Design review of the part built by this model. Coordinates are the model's own, in mm. Face numbers are marked on the shaded views. Give positions to 0.01 mm unless a question says otherwise; leave off trailing zeros. Order: outer loops, then holes, each group sorted by start corner. A loop starts at its lowest first (then second) coordinate and runs counter-clockwise, first axis right, second up. Notation, with made-up numbers: (66, 25.5) -> (102, 25.5) arc R9 cw to (102, 36.5) -> close; hole circle Ø8 at (10, 1.25). An arc over 180 degrees is marked (long way). One line per item, written item: value.
from build123d import *

# Parameters (mm, degrees)
F1_DEPTH = 25
F2_R     = 6
F2_R_2   = 8.25
F3_DEPTH = 20


with BuildPart() as f1:
    # F0 (on Top) → F1 (new body)
    with BuildSketch(Plane.XY):
        with BuildLine():
            Line((-58.75, -42.5), (58.75, -42.5))
            ThreePointArc((58.75, -42.5), (62.285534, -41.035534), (63.75, -37.5))
            Line((63.75, -37.5), (63.75, 37.5))
            ThreePointArc((63.75, 37.5), (62.285534, 41.035534), (58.75, 42.5))
            Line((58.75, 42.5), (-58.75, 42.5))
            ThreePointArc((-58.75, 42.5), (-62.285534, 41.035534), (-63.75, 37.5))
            Line((-63.75, 37.5), (-63.75, -37.5))
            ThreePointArc((-63.75, -37.5), (-62.285534, -41.035534), (-58.75, -42.5))
        make_face()
    extrude(amount=F1_DEPTH)

    # F2 (on face) → F3 (cut)
    with BuildSketch(Plane.XY.offset(25)):
        with Locations((-52.5, 15)):
            Circle(F2_R)
        with Locations((-52.5, 0)):
            Circle(F2_R)
        with Locations((-52.5, -15)):
            Circle(F2_R)
        with Locations((-37.5, 30)):
            Circle(F2_R)
        with Locations((-37.5, 15)):
            Circle(F2_R)
        with Locations((-37.5, 0)):
            Circle(F2_R)
        with Locations((-37.5, -15)):
            Circle(F2_R)
        with Locations((-37.5, -30)):
            Circle(F2_R)
        with Locations((-22.5, 30)):
            Circle(F2_R)
        with Locations((-22.5, 15)):
            Circle(F2_R)
        with Locations((-22.5, 0)):
            Circle(F2_R)
        with Locations((-22.5, -15)):
            Circle(F2_R)
        with Locations((-22.5, -30)):
            Circle(F2_R)
        with Locations((-7.5, 30)):
            Circle(F2_R)
        with Locations((-7.5, 15)):
            Circle(F2_R)
        with Locations((-7.5, 0)):
            Circle(F2_R)
        with Locations((-7.5, -15)):
            Circle(F2_R)
        with Locations((-7.5, -30)):
            Circle(F2_R)
        with Locations((7.5, 30)):
            Circle(F2_R)
        with Locations((7.5, 15)):
            Circle(F2_R)
        with Locations((7.5, 0)):
            Circle(F2_R)
        with Locations((7.5, -15)):
            Circle(F2_R)
        with Locations((7.5, -30)):
            Circle(F2_R)
        with Locations((22.5, 30)):
            Circle(F2_R)
        with Locations((22.5, 15)):
            Circle(F2_R)
        with Locations((22.5, 0)):
            Circle(F2_R)
        with Locations((22.5, -15)):
            Circle(F2_R)
        with Locations((22.5, -30)):
            Circle(F2_R)
        with Locations((37.5, 30)):
            Circle(F2_R)
        with Locations((37.5, 15)):
            Circle(F2_R)
        with Locations((37.5, 0)):
            Circle(F2_R)
        with Locations((37.5, -15)):
            Circle(F2_R)
        with Locations((37.5, -30)):
            Circle(F2_R)
        with Locations((52.5, 15)):
            Circle(F2_R)
        with Locations((52.5, 0)):
            Circle(F2_R)
        with Locations((52.5, -15)):
            Circle(F2_R)
        with Locations((-52.5, 30)):
            Circle(F2_R_2)
        with Locations((-52.5, -30)):
            Circle(F2_R_2)
        with Locations((52.5, 30)):
            Circle(F2_R_2)
        with Locations((52.5, -30)):
            Circle(F2_R_2)
    extrude(amount=-F3_DEPTH, mode=Mode.SUBTRACT)


solid = f1.part
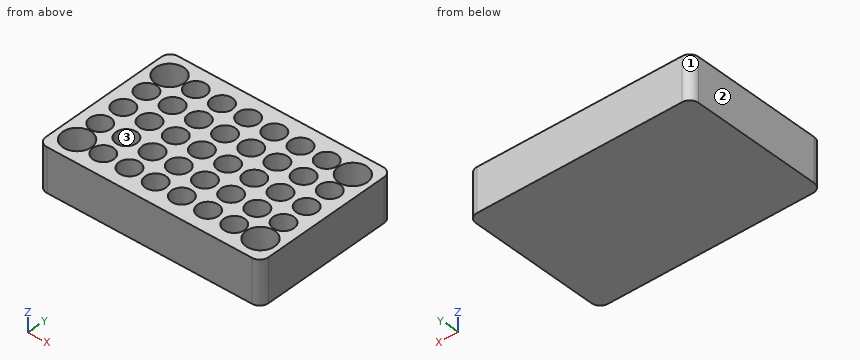
Item 1: To check wall thickness, follow line 1 along Y through (x, z) = (-37.5, 14); line 2 along Y through (x, z) = (-54, 22.25); line 3 along Z through (x, y) = (52, 27). State the ranges of each line that lie inside material, in increasing order. Write a range as from..to.
Returned:
line 1: -42.5..-36, -24..-21, -9..-6, 6..9, 21..24, 36..42.5
line 2: -42.5..-38.11, -21.89..-20.81, -9.19..-5.81, 5.81..9.19, 20.81..21.89, 38.11..42.5
line 3: 0..5
Item 2: Add section C-C on x = 52.5. Give the boundary of the cut face in (y, z).
Returned:
outline: (-42.5, 0) -> (42.5, 0) -> (42.5, 25) -> (38.25, 25) -> (38.25, 5) -> (21.75, 5) -> (21.75, 25) -> (21, 25) -> (21, 5) -> (9, 5) -> (9, 25) -> (6, 25) -> (6, 5) -> (-6, 5) -> (-6, 25) -> (-9, 25) -> (-9, 5) -> (-21, 5) -> (-21, 25) -> (-21.75, 25) -> (-21.75, 5) -> (-38.25, 5) -> (-38.25, 25) -> (-42.5, 25) -> close
Item 3: Add section A-A on x = 22.5. Give the boundary of the cut face in (y, z).
Returned:
outline: (-42.5, 0) -> (42.5, 0) -> (42.5, 25) -> (36, 25) -> (36, 5) -> (24, 5) -> (24, 25) -> (21, 25) -> (21, 5) -> (9, 5) -> (9, 25) -> (6, 25) -> (6, 5) -> (-6, 5) -> (-6, 25) -> (-9, 25) -> (-9, 5) -> (-21, 5) -> (-21, 25) -> (-24, 25) -> (-24, 5) -> (-36, 5) -> (-36, 25) -> (-42.5, 25) -> close
Item 4: Clearance check with flat-ended pins moving along their axes: P1, Ø13, axis at x = -38, y = -15.5, coming from the +Z side; P2, Ø3.5, axis at x = -50, y = 13, coming from the +Z side. State where each tip first meets the part, or that it passes through.
Returned:
P1: z = 25
P2: z = 5
Item 5: Draft analysis for pull direction Y (two halves, no side actions). For the marked faces 1, 2 and 3, state which applies: pulls with the +Y half, pulls with the -Y half, needs draft (parallel to the pull), parting line crosses it, or undercut.
Returned:
face 1: pulls with the +Y half
face 2: needs draft
face 3: undercut
Item 6: Add section B-B on z = 16. Count the separate pieces of the cut face and the enclosed holes in it, plus the area to 3 significant figures.
Returned:
separate pieces: 1
enclosed holes: 40
area: 5,890 mm²
